```python
from build123d import *

# Parameters (mm, degrees)
BOSS_EXTRUDE2_DEPTH = 1.5748


with BuildPart() as part:
    # Sketch1 → Boss-Extrude2 (new body)
    with BuildSketch(Plane(origin=(0, 0, 0), x_dir=(1, 0, 0), z_dir=(0, 1, 0))):
        with BuildLine():
            ThreePointArc((105.621971622, 137.184472252), (31.75, 323.85), (-42.121971622, 137.184472252))
            Line((-42.121971622, 137.184472252), (-45.184156549, 133.7228719))
            ThreePointArc((-45.184156549, 133.7228719), (-222.25, 50.8), (-45.184156549, -32.1228719))
            Line((-45.184156549, -32.1228719), (-42.121971622, -35.584472252))
            ThreePointArc((-42.121971622, -35.584472252), (31.75, -222.25), (105.621971622, -35.584472252))
            Line((105.621971622, -35.584472252), (108.684156549, -32.1228719))
            ThreePointArc((108.684156549, -32.1228719), (285.75, 50.8), (108.684156549, 133.7228719))
            Line((108.684156549, 133.7228719), (105.621971622, 137.184472252))
        make_face()
        with BuildLine():
            ThreePointArc((19.066089569, -104.753584904), (16.904555213, -119.923912703), (28.575, -129.854259867))
            Line((28.575, -129.854259867), (28.575, -215.850378507))
            ThreePointArc((28.575, -215.850378507), (-63.260846634, -150.293041299), (-37.912692613, -40.342787654))
            Line((-37.912692613, -40.342787654), (19.066089569, -104.753584904))
        make_face(mode=Mode.SUBTRACT)
        with BuildLine():
            Line((-215.850378507, 47.625), (-129.854259867, 47.625))
            ThreePointArc((-129.854259867, 47.625), (-120.820607869, 36.325978513), (-106.372217741, 37.046240752))
            Line((-106.372217741, 37.046240752), (-49.393435559, -27.364556498))
            ThreePointArc((-49.393435559, -27.364556498), (-156.031890363, -41.833737519), (-215.850378507, 47.625))
        make_face(mode=Mode.SUBTRACT)
        with BuildLine():
            Line((-101.616089569, 60.346415096), (-44.637307387, 124.757212346))
            ThreePointArc((-44.637307387, 124.757212346), (-12.7, 50.8), (-44.637307387, -23.157212346))
            Line((-44.637307387, -23.157212346), (-101.616089569, 41.253584904))
            ThreePointArc((-101.616089569, 41.253584904), (-98.425, 50.8), (-101.616089569, 60.346415096))
        make_face(mode=Mode.SUBTRACT)
        with BuildLine():
            Line((44.433910431, -104.753584904), (101.412692613, -40.342787654))
            ThreePointArc((101.412692613, -40.342787654), (126.760846634, -150.293041299), (34.925, -215.850378507))
            Line((34.925, -215.850378507), (34.925, -129.854259867))
            ThreePointArc((34.925, -129.854259867), (46.595444787, -119.923912703), (44.433910431, -104.753584904))
        make_face(mode=Mode.SUBTRACT)
        with BuildLine():
            ThreePointArc((-33.156564441, -36.135443502), (31.75, -12.7), (96.656564441, -36.135443502))
            Line((96.656564441, -36.135443502), (39.677782259, -100.546240752))
            ThreePointArc((39.677782259, -100.546240752), (31.75, -98.425), (23.822217741, -100.546240752))
            Line((23.822217741, -100.546240752), (-33.156564441, -36.135443502))
        make_face(mode=Mode.SUBTRACT)
        with BuildLine():
            ThreePointArc((108.137307387, -23.157212346), (76.2, 50.8), (108.137307387, 124.757212346))
            Line((108.137307387, 124.757212346), (165.116089569, 60.346415096))
            ThreePointArc((165.116089569, 60.346415096), (161.925, 50.8), (165.116089569, 41.253584904))
            Line((165.116089569, 41.253584904), (108.137307387, -23.157212346))
        make_face(mode=Mode.SUBTRACT)
        with BuildLine():
            ThreePointArc((169.872217741, 37.046240752), (184.320607869, 36.325978513), (193.354259867, 47.625))
            Line((193.354259867, 47.625), (279.350378507, 47.625))
            ThreePointArc((279.350378507, 47.625), (219.531890363, -41.833737519), (112.893435559, -27.364556498))
            Line((112.893435559, -27.364556498), (169.872217741, 37.046240752))
        make_face(mode=Mode.SUBTRACT)
        with BuildLine():
            ThreePointArc((-215.850378507, 53.975), (-156.031890363, 143.433737519), (-49.393435559, 128.964556498))
            Line((-49.393435559, 128.964556498), (-106.372217741, 64.553759248))
            ThreePointArc((-106.372217741, 64.553759248), (-120.820607869, 65.274021487), (-129.854259867, 53.975))
            Line((-129.854259867, 53.975), (-215.850378507, 53.975))
        make_face(mode=Mode.SUBTRACT)
        with BuildLine():
            Line((28.575, 317.450378507), (28.575, 231.454259867))
            ThreePointArc((28.575, 231.454259867), (16.904555213, 221.523912703), (19.066089569, 206.353584904))
            Line((19.066089569, 206.353584904), (-37.912692613, 141.942787654))
            ThreePointArc((-37.912692613, 141.942787654), (-63.260846634, 251.893041299), (28.575, 317.450378507))
        make_face(mode=Mode.SUBTRACT)
        with BuildLine():
            Line((-33.156564441, 137.735443502), (23.822217741, 202.146240752))
            ThreePointArc((23.822217741, 202.146240752), (31.75, 200.025), (39.677782259, 202.146240752))
            Line((39.677782259, 202.146240752), (96.656564441, 137.735443502))
            ThreePointArc((96.656564441, 137.735443502), (31.75, 114.3), (-33.156564441, 137.735443502))
        make_face(mode=Mode.SUBTRACT)
        with BuildLine():
            Line((279.350378507, 53.975), (193.354259867, 53.975))
            ThreePointArc((193.354259867, 53.975), (184.320607869, 65.274021487), (169.872217741, 64.553759248))
            Line((169.872217741, 64.553759248), (112.893435559, 128.964556498))
            ThreePointArc((112.893435559, 128.964556498), (219.531890363, 143.433737519), (279.350378507, 53.975))
        make_face(mode=Mode.SUBTRACT)
        with BuildLine():
            ThreePointArc((44.433910431, 206.353584904), (46.595444787, 221.523912703), (34.925, 231.454259867))
            Line((34.925, 231.454259867), (34.925, 317.450378507))
            ThreePointArc((34.925, 317.450378507), (126.760846634, 251.893041299), (101.412692613, 141.942787654))
            Line((101.412692613, 141.942787654), (44.433910431, 206.353584904))
        make_face(mode=Mode.SUBTRACT)
    extrude(amount=BOSS_EXTRUDE2_DEPTH)


solid = part.part
```
Can you work these out from the model? Positions are in its coordinate system, mm. Coordinates: 2 decimals unless noted, no trailing zeros. Loops run counter-clockwise (first coordinate to the right, second up) from the corner with the lowest first, then second, coordinate; pieces in that order, holes last.
Item 1: Suppose I cut it at D-D (y = 0.6). State how many separate pieces and enclosed holes the cut face has, then the cut area to 3 significant figures.
Answers below:
separate pieces: 1
enclosed holes: 12
area: 38,100 mm2
Item 2: Please list where these lines run through material, in increasing order: L1, parallel to X at y = 0.85, z = -58.5; L2, parallel to X at y = 0.5, z = 167.5 (3 decimals); L3, parallel to X at y = 1.15, z = 165.5 (3 decimals).
Answers below:
L1: x = -221.98 to -215.61, -128.18 to -100.42, -12.99 to 76.49, 163.92 to 191.68, 279.11 to 285.48
L2: x = -62.181 to -54.808, 28.575 to 34.925, 118.308 to 125.681
L3: x = -63.286 to -56.006, 28.575 to 34.925, 119.506 to 126.786
Item 3: If we mould it in two halves opening along X, with no side actions, what happens to faces 1 (the face through (31, 0, -32)), 2 (the face through (-120.63, 0.78, -65.36)), 3 (the face through (-62.655, 0.776, 151.854))? For each: released by +X, released by -X, zero draft, split by the parting line, or undercut.
Answers below:
face 1: zero draft
face 2: undercut
face 3: undercut
Item 4: Suppose I cut it at C-C (x = 58). Please give me the cut outline in (y, z).
Answers below:
outline: (0, -320.61) - (1.57, -320.61) - (1.57, -314.05) - (0, -314.05) - close; (0, -191.02) - (1.57, -191.02) - (1.57, -181.43) - (0, -181.43) - close; (0, -117.75) - (1.57, -117.75) - (1.57, 16.15) - (0, 16.15) - close; (0, 79.83) - (1.57, 79.83) - (1.57, 89.42) - (0, 89.42) - close; (0, 212.45) - (1.57, 212.45) - (1.57, 219.01) - (0, 219.01) - close
Item 5: I'm going to push flat-ended pins straight in: pin 1 (0.5 mm diameter, centred on x = 237, y = 1, fed in from +Z); pin 2 (0.8 mm diameter, centred on y = 1, z = 170, fed in from +X); pin 3 (0.8 mm diameter, centred on y = 0.5, z = 183.5, fed in from -X). Where does each tip first touch, or does it pass through?
Answers below:
pin 1: stops at z = 39.63
pin 2: stops at x = 124.46
pin 3: stops at x = -51.44
Item 6: Suppose I cut it at B-B (z = -215.9). Please give me the cut outline in (x, y) (3 decimals), then the cut area to 3 significant figures.
Answers below:
outline: (-76.2, 0) - (-69.85, 0) - (-69.85, 1.575) - (-76.2, 1.575) - close; (15.875, 0) - (47.625, 0) - (47.625, 1.575) - (15.875, 1.575) - close; (133.35, 0) - (139.7, 0) - (139.7, 1.575) - (133.35, 1.575) - close
area: 70.0 mm2
Item 7: Suppose I cut it at A-A (x = 177.8). Please give me the cut outline in (y, z) (3 decimals), then the cut area to 3 significant figures.
Answers below:
outline: (0, -158.75) - (1.575, -158.75) - (1.575, -152.4) - (0, -152.4) - close; (0, -66.675) - (1.575, -66.675) - (1.575, -34.925) - (0, -34.925) - close; (0, 50.8) - (1.575, 50.8) - (1.575, 57.15) - (0, 57.15) - close
area: 70.0 mm2
